Build history of the part. All positions in model axes, mm. A direction names the side the tool comes from. Coordinates: 2 decimals unless noted, no trailing zeros. Write each loop counter-clockwise with the first axis right and the second up, starting at its lowest first coordinate (ties: lowest second). Pieces come first, ordered by that corner, then holes.
Autodesk Inventor part; units mm, degrees
ref_plane "YZ Plane" through (0, 0, 0) normal (1, 0, 0) x (0, 1, 0)
ref_plane "XZ Plane" through (0, 0, 0) normal (0, 1, 0) x (-1, 0, 0)
ref_plane "XY Plane" through (0, 0, 0) normal (0, 0, 1) x (1, 0, 0)
sketch "Sketch1" plane through (0, 0, 0) normal (0, 0, 1) x (1, 0, 0)
  line L0 (0, 0) -> (160, 0)
  line L1 (160, 0) -> (118.589, -154.5481)
  line L2 (0, 0) -> (41.411, -154.5481)
  line L3 (41.411, -154.5481) -> (118.589, -154.5481)
  dimension "d4" = 160
  dimension "d5" = 160
  dimension "d6" = 160
  dimension "d7" = 75
extrude "Extrusion1" add sketch "Sketch1" along normal blind 415
sketch "Sketch2" plane through (0, 0, 415) normal (0, 0, 1) x (1, 0, 0)
  circle A0 centre (235.8871, -103.156) radius 80 construction
  circle A1 centre (-75.8871, -103.156) radius 80 construction
  line L0 (160, 0) -> (0, 0)
  line L1 (-96.5926, -25.8819) -> (0, 0)
  line L2 (0, 0) -> (41.411, -154.5481)
  line L3 (-55.1815, -180.43) -> (41.411, -154.5481)
  line L4 (0, 0) -> (41.411, -154.5481)
  arc A2 (-96.5926, -25.8819) -> (-55.1815, -180.43) centre (-75.8871, -103.156) ccw
  line L5 (41.411, -154.5481) -> (118.589, -154.5481)
  line L6 (118.589, -154.5481) -> (215.1815, -180.43)
  line L7 (160, 0) -> (256.5926, -25.8819)
  arc A3 (215.1815, -180.43) -> (256.5926, -25.8819) centre (235.8871, -103.156) ccw
  line L8 (160, 0) -> (118.589, -154.5481)
  dimension "d8" = 160
  dimension "d9" = 160
  dimension "d10" = 100
  dimension "d13" = 100
extrude "Extrusion2" add sketch "Sketch2" against normal blind 415 contours L7 A3 L6 L8 | L2 L3 A2 L1
properties part number "CA003" material "ABS Plastic"
1. Saw through at A-A on z = 133.5. List the corners of the cut face in (x, y), plus the area to 3 significant figures.
Computed values:
outline: (-96.59, -25.88) arc R80 ccw to (-55.18, -180.43) - (41.41, -154.55) - (118.59, -154.55) - (215.18, -180.43) arc R80 ccw to (256.59, -25.88) - (160, 0) - (0, 0) - close
area: 70,400 mm2
2. Saw through at B-B on y = -132. List the corners of the cut face in (x, z), plus the area to 3 significant figures.
Computed values:
outline: (-150.51, 0) - (310.51, 0) - (310.51, 415) - (-150.51, 415) - close
area: 191,000 mm2
3. Flat gauge pins, fed straight in: pin 1 (1.5 mm diameter, centred on x = 147.5, z = 369.5, fed in from -Y); pin 2 (1 mm diameter, centred on x = -96.5, z = 360, fed in from +Y); pin 3 (8 mm diameter, centred on y = -28, z = 318.5, fed in from +X). Where does each tip first touch, or does it go through?
Computed values:
pin 1: stops at y = -162.5
pin 2: stops at y = -25.72
pin 3: stops at x = 272.45
4. Probe line 1 along Y through (x, z) = (59.5, 336.5); line 2 along Y through (x, z) = (34.5, 226); line 3 along X through (y, z) = (-154, 42). List the from-to ranges inside material, lowest first.
Computed values:
line 1: y = -154.55 to 0
line 2: y = -156.4 to 0
line 3: x = -137.65 to 297.65
5. Saw through at C-C on x = 225.5. List the corners of the cut face in (y, z), plus the area to 3 significant figures.
Computed values:
outline: (-182.48, 0) - (-17.55, 0) - (-17.55, 415) - (-182.48, 415) - close
area: 68,400 mm2
6. Mould opens along X. For faces 1 (the face through (79, -154.548, 205)), 2 (the face through (-48.97, -13.12, 210.4)), 3 (the face through (79, 0, 205)) say: +X half, -X half, draft (parallel to the pull), parting line (faces both ways), or undercut.
Computed values:
face 1: undercut
face 2: -X half
face 3: draft
7. 3-axis set-ups, long thin cutter, end or side, ignore diameter. For faces 4 (the face through (77, -90, 415)), 5 (the face through (166.21, -167.31, 210.4)): which of +Z, -Z, +X, -X, +Y, -Y reach the whole face in a straight line?
Computed values:
face 4: +Z, +X, -X, +Y, -Y
face 5: +Z, -Z, -Y
